Autodesk Fusion 360 part; units mm, degrees
sketch "Sketch1" plane through (0, 0, 0) normal (0, 0, 1) x (1, 0, 0)
  circle A0 centre (0, 0) radius 6
  circle A1 centre (0, 0) radius 8.5
  circle A2 centre (0, 0) radius 2.5
  dimension "d1" = 12
  dimension "d2" = 17
  dimension "d3" = 5
extrude "Extrude1" add sketch "Sketch1" along normal blind 6.5 contours A0
extrude "Extrude2" add sketch "Sketch1" against normal blind 1 contours A0 | A1
sketch "Sketch2" plane through (0, 0, 6.5) normal (0, 0, 1) x (-1, 0, 0)
  circle A0 centre (0, 0) radius 2.5
  circle A1 centre (0, 0) radius 6
  circle A2 centre (0, 0) radius 8.5
  dimension "d8" = 17
extrude "Extrude3" add sketch "Sketch2" along normal blind 1 contours A1 | A2
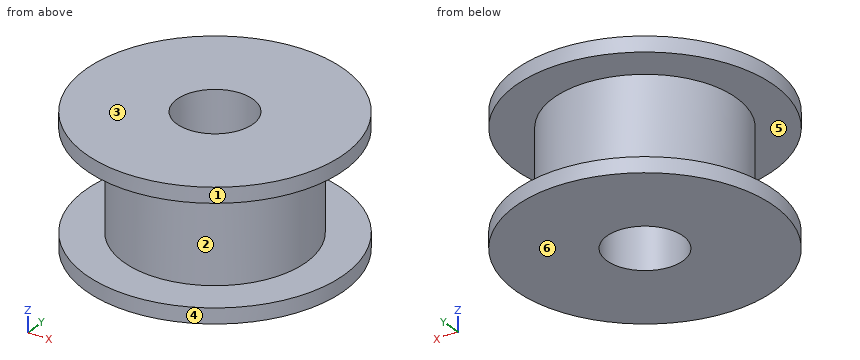
The listing builds one solid part. Answer for the finished solid, in the listing's coordinates (mm). Face numbers are marked on the shaded views. A direction names the side the tool comes from. Coordinates: 2 decimals unless noted, no trailing zeros. Write each loop counter-clockwise with the first axis right and the second up, starting at its lowest first coordinate (ties: lowest second). Pieces come first, ordered by that corner, then holes. Notation, with made-up numbers: (51, 88) - (85, 88) arc R22 ccw to (85, 118) - close; hole circle Ø5 at (59, -7). An arc over 180 degrees is marked (long way). Return JSON: item names as keys, results as strings. Group by question number.
Q1. The part is cut by section D-D on y = -4. Write down the section's boundary in (x, z).
Q2. Find the intervals of material crossed by line 1 along Z through (x, y) = (-6.5, -3.75); line 2 along Y through (x, z) = (0, 3.25); line 3 along X through (y, z) = (-2, 5.75), in increasing order. Write a range as [from, to].
Q3. For a pull along Z with two mould halves and no side action, classify the marked faces 3, 4, 5 and 6 as +Z half, -Z half, draft (parallel to the pull), parting line (faces both ways), or undercut.
Q4. The part is cut by section B-B on y = -1. Write down the section's boundary in (x, z).
Q5. Which of the six approach directions +Z, -Z, +X, -X, +Y, -Y give full straight-line access (tool end or side, diameter ignored) to the marked faces 1 and 2?
Q6. The part is cut by section C-C on z = 3. Write down the section's boundary in (x, y).
Evaluation:
{
 "1": {"outline": "(-7.5, -1) - (7.5, -1) - (7.5, 0) - (4.47, 0) - (4.47, 6.5) - (7.5, 6.5) - (7.5, 7.5) - (-7.5, 7.5) - (-7.5, 6.5) - (-4.47, 6.5) - (-4.47, 0) - (-7.5, 0) - close"},
 "2": {"line 1": "z = [-1, 0], [6.5, 7.5]", "line 2": "y = [-6, -2.5], [2.5, 6]", "line 3": "x = [-5.66, -1.5], [1.5, 5.66]"},
 "3": {"face 3": "+Z half", "face 4": "draft", "face 5": "undercut", "face 6": "-Z half"},
 "4": {"outline": "(-8.44, -1) - (-2.29, -1) - (-2.29, 7.5) - (-8.44, 7.5) - (-8.44, 6.5) - (-5.92, 6.5) - (-5.92, 0) - (-8.44, 0) - close; (2.29, -1) - (8.44, -1) - (8.44, 0) - (5.92, 0) - (5.92, 6.5) - (8.44, 6.5) - (8.44, 7.5) - (2.29, 7.5) - close"},
 "5": {"face 1": "+Z, -Z", "face 2": "none"},
 "6": {"outline": "circle Ø12 at (0, 0); hole circle Ø5 at (0, 0)"}
}
